Autodesk Inventor part; units mm, degrees
ref_plane "YZ Plane" through (0, 0, 0) normal (1, 0, 0) x (0, 1, 0)
ref_plane "XZ Plane" through (0, 0, 0) normal (0, 1, 0) x (-1, 0, 0)
ref_plane "XY Plane" through (0, 0, 0) normal (0, 0, 1) x (1, 0, 0)
sketch "Эскиз1" plane through (0, 0, 0) normal (0, 0, 1) x (1, 0, 0)
  circle A0 centre (-7.5, -22.95) radius 1.5
  circle A1 centre (7.5, -22.95) radius 1.5
  circle A2 centre (7.5, -6.95) radius 1.5
  circle A3 centre (-7.5, -6.95) radius 1.5
  line L0 (-281.4, 13.05) -> (10, 13.05)
  line L1 (10, 13.05) -> (10, -42.95)
  line L2 (10, -42.95) -> (-281.4, -42.95)
  line L3 (-281.4, -42.95) -> (-281.4, 13.05)
  line L4 (-281.4, 13.05) -> (10, -42.95) construction
  line L5 (10, 13.05) -> (-281.4, -42.95) construction
  line L6 (-135.7, -14.95) -> (-135.7, -42.95) construction
  circle A4 centre (-263.9, -22.95) radius 1.5
  circle A5 centre (-278.9, -22.95) radius 1.5
  circle A6 centre (-278.9, -6.95) radius 1.5
  circle A7 centre (-263.9, -6.95) radius 1.5
  point P0 (0, 0)
  dimension "d5" = 291.4
  dimension "d8" = 2.5
  dimension "d9" = 20
  dimension "d10" = 20
extrude "Выдавливание1" add sketch "Эскиз1" along normal blind 4
sketch "Эскиз3" plane through (0, 0, 4) normal (0, 0, 1) x (1, 0, 0)
  line L0 (-281.4, -42.95) -> (10, -42.95) construction
  line L1 (10, 13.05) -> (-281.4, 13.05) construction
  circle A0 centre (-257.7118, -2.95) radius 2.6
  circle A1 centre (-257.5855, -26.9497) radius 2.6
  line L2 (10, -39.95) -> (-281.4, -39.95) construction
  line L3 (-281.4, 10.05) -> (10, 10.05) construction
  line L4 (-135.7, -39.95) -> (-135.7, 10.05) construction
  circle A2 centre (-13.6882, -2.95) radius 2.6
  circle A3 centre (-13.8145, -26.9497) radius 2.6
  point P0 (0, 0)
extrude "Выдавливание2" cut sketch "Эскиз3" against normal blind 4
sketch "Эскиз4" plane through (0, 0, 0) normal (0, 0, -1) x (-1, 0, 0)
  line L0 (27.7, 29.05) -> (243.7, 29.05)
  line L1 (243.7, 29.05) -> (243.7, -2.95)
  line L2 (243.7, -2.95) -> (27.7, -2.95)
  line L3 (27.7, -2.95) -> (27.7, 29.05)
  line L4 (-10, 13.05) -> (281.4, 13.05)
  line L5 (27.7, 29.05) -> (243.7, -2.95) construction
  line L6 (243.7, 29.05) -> (27.7, -2.95) construction
  point P0 (0, 0)
  point P1 (135.7, 13.05)
  point P2 (243.7, 13.05)
  dimension "d13" = 16
  dimension "d14" = 216
extrude "Выдавливание3" cut sketch "Эскиз4" against normal blind 4
ref_plane "РабПлоскость1" through (-281.4, -14.95, 0) normal (0, -1, 0) x (1, 0, 0)
mirror "Зеркальное отражение1" about plane through (-281.4, -14.95, 0) normal (0, -1, 0) of "Выдавливание3"
sketch "Эскиз5" plane through (0, 0, 4) normal (0, 0, 1) x (1, 0, 0)
  circle A0 centre (4.7234, -38.95) radius 1.25
  circle A1 centre (-4.7766, -38.95) radius 1.25
  line L0 (-243.7, -26.95) -> (-27.7, -26.95)
  line L1 (-135.7, -26.95) -> (-135.7, -2.95)
  line L2 (-243.7, -2.95) -> (-27.7, -2.95)
  circle A2 centre (-276.1234, -36.95) radius 1.25
  circle A3 centre (-266.6234, -36.95) radius 1.25
  line L3 (-27.7, -42.95) -> (10, -42.95)
  point P0 (0, 0)
  dimension "d23" = 4
  dimension "d25" = 2.5
  dimension "d26" = 2.5
  dimension "d27" = 4
  dimension "d28" = 9.5
extrude "Выдавливание4" cut sketch "Эскиз5" against normal blind 10
sketch "Эскиз7" plane through (0, 0, 4) normal (0, 0, 1) x (1, 0, 0)
  circle A0 centre (-20, -14.95) radius 1.6
  circle A1 centre (-65.7, -14.95) radius 1.6
  line L0 (-243.7, -2.95) -> (-27.7, -2.95)
  line L1 (-135.7, -2.95) -> (-135.7, -16.103)
  circle A2 centre (-251.4, -14.95) radius 1.6
  circle A3 centre (-205.7, -14.95) radius 1.6
  line L2 (10, -42.95) -> (10, 13.05)
  line L3 (10, -14.95) -> (-93.8344, -14.95)
  point P0 (0, 0)
  dimension "d29" = 45.7
  dimension "d30" = 3.2
  dimension "d31" = 3.2
  dimension "d32" = 30
extrude "Выдавливание6" cut sketch "Эскиз7" against normal blind 10
properties part number "центр_рейка" material "Древесина (береза)"
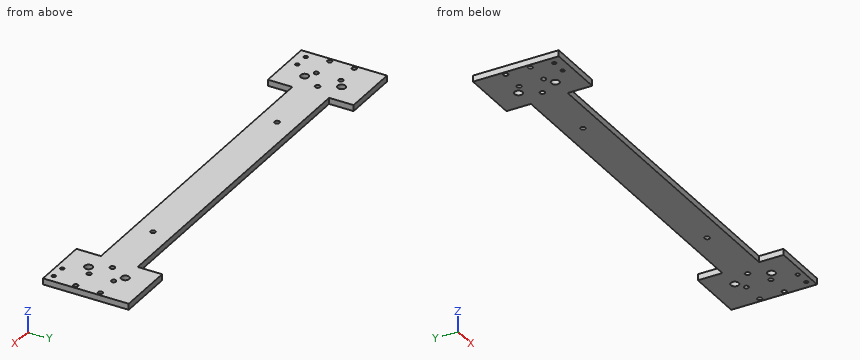
Part model, mm, in its own coordinate system. Round coordinates to 2 decimals unless told otherwise and drop trailing zeros. Write each loop counter-clockwise with the first axis right and the second up, starting at its lowest first coordinate (ties: lowest second). Pieces come first, ordered by that corner, then holes. Notation, with made-up numbers: M 57.25,5 L 65.25,5 A27 cw 65.25,37 Z; hole C -32.75,56.5 d1. An arc over 180 degrees is marked long. Answer as CSV lines item,"result". Start each with the question number.
1) Drill centre lines: L1, parallel to X at y = -3.5, z = 2.5; L2, parallel to X at y = -27.5, z = 0.65; L3, parallel to X at y = 1, z = 3.2. Where is each one in solid material? Low to high.
2) Band-saw the part on A-A (z = 2.05). Count the separate pieces of the cut face and the enclosed holes in it, then the cut area to 3 significant figures.
3) Band-saw the part on B-B (x = -91.5). List the corners of the cut face in (y, z), then the cut area to 3 significant figures.
4) Drop flat-ended pins along their axis: pin 1 (2 mm diameter, centred on x = -36.5, z = 1, fed in from -Y); pin 2 (8.5 mm diameter, centred on x = -13.69, y = -2.95, fed in from -Z). Give the stop position or say it passes through.
Worked out:
1,L1,"-281.4 to -260.25, -255.17 to -16.23, -11.15 to 10"
1,L2,"-281.4 to -260.13, -255.04 to -243.7, -27.7 to -16.36, -11.27 to 10"
1,L3,"-281.4 to -243.7, -27.7 to 10"
2,separate pieces,"1"
2,enclosed holes,"20"
2,area,"9,210 mm²"
3,outline,"M -26.95,0 L -2.95,0 L -2.95,4 L -26.95,4 Z"
3,area,"96.0 mm²"
4,pin 1,"y = -26.95"
4,pin 2,"z = 0"
